Work out the finished part from the listing and answer in its coordinate system (mm). A direction names the side the tool comes from. Round coordinates to 2 decimals unless told otherwise and drop trailing zeros. Write each loop counter-clockwise with the first axis right and the second up, starting at its lowest first coordinate (ties: lowest second). Pieces come first, ordered by that corner, then holes. Notation, with made-up numbers: M 12,0 L 47,0 A25 ccw 47,34 Z; hole C -17,5 d6. An arc over 180 degrees is marked long. Answer in a Markdown table with one row per item.
```python
from build123d import *

# Parameters (mm, degrees)
D_GAGEMENT_M81_D                              = 9
D_GAGEMENT_M81_DEPTH                          = 13.8
TROU_POUR_TARAUDAGE_POUR_TROU_TARAUD_M4_REACH = 26.576
TROU_POUR_TARAUDAGE_POUR_TROU_TARAUD_2_R      = 1.65
TROU_POUR_TARAUDAGE_POUR_TROU_TARAUD_M3_D     = 2.5
TROU_POUR_TARAUDAGE_POUR_TROU_TARAUD_M3_DEPTH = 5


with BuildPart() as part:
    # Esquisse1 → Révolution1 (revolve)
    with BuildSketch(Plane.XY, mode=Mode.PRIVATE) as r_volution1_sk:
        Polygon((0, 0), (0, 7), (0.8, 7), (0.8, 9), (8.8, 9), (8.8, 15.5), (13.8, 15.5), (13.8, 0), align=None)
    revolve(r_volution1_sk.sketch.rotate(Axis((0, 0, 0), (1, 0, 0)), 90), axis=Axis((0, 0, 0), (1, 0, 0)))  # turned: the seam where the file's is

    # Dégagement M81
    with Locations(Plane.ZY):
        with Locations((0, 0)):
            Hole(D_GAGEMENT_M81_D / 2, depth=D_GAGEMENT_M81_DEPTH)

    # Trou pour taraudage pour trou taraud 2 (on position points) → Trou pour taraudage pour trou taraudé M4x0.71 (cut, up to next)
    with BuildSketch(Plane(origin=(4.566426523, 0.044478819, -8.99989009), x_dir=(0, -0.999987788, -0.004942091), z_dir=(0, 0.004942091, -0.999987788)), mode=Mode.PRIVATE) as trou_pour_taraudage_pour_trou_taraud_m4_sk1:
        Circle(TROU_POUR_TARAUDAGE_POUR_TROU_TARAUD_2_R)
    trou_pour_taraudage_pour_trou_taraud_m4_tool1 = extrude(trou_pour_taraudage_pour_trou_taraud_m4_sk1.sketch, amount=-TROU_POUR_TARAUDAGE_POUR_TROU_TARAUD_M4_REACH, mode=Mode.PRIVATE) & part.part
    add(trou_pour_taraudage_pour_trou_taraud_m4_tool1.solids().sort_by_distance((4.566427, 0.044479, -8.99989))[0], mode=Mode.SUBTRACT)

    # Trou pour taraudage pour trou taraudé M3x0.51
    with Locations(Plane.ZY.offset(-8.8)):
        with Locations((-10.718944801, 7.355557243), (7.174803364, 10.840765503), (10.695756801, -7.389234497), (-7.534243199, -10.594110601)):
            Hole(TROU_POUR_TARAUDAGE_POUR_TROU_TARAUD_M3_D / 2, depth=TROU_POUR_TARAUDAGE_POUR_TROU_TARAUD_M3_DEPTH)


solid = part.part
```
1. The part is cut by section A-A (z = 0). Determine the outline of the cut face in (x, y).
Calculated:
| item | result |
|---|---|
| outline | M 0,-7 L 0.8,-7 L 0.8,-9 L 8.8,-9 L 8.8,-15.5 L 13.8,-15.5 L 13.8,-4.5 L 0,-4.5 Z; M 0,4.5 L 13.8,4.5 L 13.8,15.5 L 8.8,15.5 L 8.8,9 L 0.8,9 L 0.8,7 L 0,7 Z |
2. A tool of negligible diameter and unlimited length cuts with its end or side. For faces 1 (the cylindrical face through (6.997, 0.198, 4.496)), 2 (the flat face through (8.8, 7, -7)), from which of +Z, -Z, +X, -X, +Y, -Y can it reach the whole face along a straight path? Write none if from no direction.
Calculated:
| item | result |
|---|---|
| face 1 | +X, -X |
| face 2 | -X |
3. The part is cut by section B-B (y = -2). Determine the outline of the cut face in (x, z), plus the area to 3 significant figures.
Calculated:
| item | result |
|---|---|
| outline | M 0,-6.71 L 0.8,-6.71 L 0.8,-8.77 L 8.8,-8.77 L 8.8,-15.37 L 13.8,-15.37 L 13.8,-4.03 L 0,-4.03 Z; M 0,4.03 L 13.8,4.03 L 13.8,15.37 L 8.8,15.37 L 8.8,8.77 L 0.8,8.77 L 0.8,6.71 L 0,6.71 Z |
| area | 194 mm² |
4. Determine the mould class of faces 3 (the cylindrical face through (11.34, -7.87, 9.54)), 4 (the flat face through (0.8, 7.3, 0)), 5 (the cylindrical face through (6.03, -0.73, -6.63)) for opening direction X: released by +X, released by -X, zero draft, split by the parting line, or undercut.
Calculated:
| item | result |
|---|---|
| face 3 | zero draft |
| face 4 | released by -X |
| face 5 | undercut |
5. Given pin 1 (2 mm diameter, centred on x = 12, z = 7.5, fed in from -Y); pin 2 (1.5 mm diameter, centred on x = 6, y = 7, fed in from -Z); pin 3 (2 mm diameter, centred on x = 9, y = 11.5, fed in from -Z); pin 4 (3 mm diameter, centred on y = 7.36, z = -10.72, fed in from +X), each flat-ended and moving along its own axis, determine where each tip first touches the part or whether it passes through.
Calculated:
| item | result |
|---|---|
| pin 1 | stops at y = -14.07 |
| pin 2 | stops at z = -6.48 |
| pin 3 | stops at z = -11.4 |
| pin 4 | stops at x = 13.8 |
6. The part is cut by section D-D (x = 10.5). Determine the outline of the cut face in (y, z).
Calculated:
| item | result |
|---|---|
| outline | C 0,0 d31; hole C -10.59,-7.53 d2.5; hole C -7.39,10.7 d2.5; hole C 0,0 d9; hole C 7.36,-10.72 d2.5; hole C 10.84,7.17 d2.5 |
7. The part is cut by section C-C (x = 7.5). Determine the outline of the cut face in (y, z).
Calculated:
| item | result |
|---|---|
| outline | C 0,0 d18; hole C 0,0 d9 |
8. Consider line 1 along Y through (x, z) = (9.75, 0); line 2 along Z through (x, y) = (1.75, -2.5); line 3 along X through (y, z) = (1.5, -10.5). Determine where each line is inside the solid, lowest interval first. Write a range as from..to.
Calculated:
| item | result |
|---|---|
| line 1 | y = -15.5..-4.5, 4.5..15.5 |
| line 2 | z = -8.65..-3.74, 3.74..8.65 |
| line 3 | x = 8.8..13.8 |
